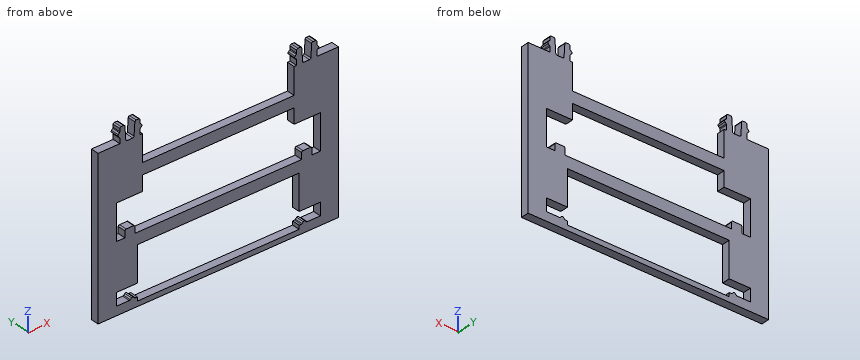
```python
from build123d import *

# Parameters (mm, degrees)
BOSS_EXTRUDE1_DEPTH = 1.6


with BuildPart() as part:
    # Sketch1 → Boss-Extrude1 (new body)
    with BuildSketch(Plane(origin=(0, 0, 0), x_dir=(1, 0, 0), z_dir=(0, 1, 0))):
        with BuildLine():
            Line((-68.929583289, 0), (-64.629583289, 0))
            Line((-64.629583289, 0), (-64.629583289, -0.996446609))
            ThreePointArc((-64.629583289, -0.996446609), (-64.648613406, -1.092117467), (-64.702806594, -1.173223305))
            Line((-64.702806594, -1.173223305), (-64.952806594, -1.423223305))
            ThreePointArc((-64.952806594, -1.423223305), (-65.026029899, -1.6), (-64.952806594, -1.776776695))
            Line((-64.952806594, -1.776776695), (-64.702806594, -2.026776695))
            ThreePointArc((-64.702806594, -2.026776695), (-64.648613406, -2.107882533), (-64.629583289, -2.203553391))
            Line((-64.629583289, -2.203553391), (-64.629583289, -2.75))
            ThreePointArc((-64.629583289, -2.75), (-64.556359984, -2.926776695), (-64.379583289, -3))
            Line((-64.379583289, -3), (-63.863471562, -3))
            ThreePointArc((-63.863471562, -3), (-63.692675541, -2.932561549), (-63.614025273, -2.766629753))
            Line((-63.614025273, -2.766629753), (-63.445141306, -0.233370247))
            ThreePointArc((-63.445141306, -0.233370247), (-63.366491038, -0.067438451), (-63.195695016, 0))
            Line((-63.195695016, 0), (-62.063471562, 0))
            ThreePointArc((-62.063471562, 0), (-61.892675541, -0.067438451), (-61.814025273, -0.233370247))
            Line((-61.814025273, -0.233370247), (-61.645141306, -2.766629753))
            ThreePointArc((-61.645141306, -2.766629753), (-61.566491038, -2.932561549), (-61.395695016, -3))
            Line((-61.395695016, -3), (-60.879583289, -3))
            ThreePointArc((-60.879583289, -3), (-60.702806594, -2.926776695), (-60.629583289, -2.75))
            Line((-60.629583289, -2.75), (-60.629583289, -2.203553391))
            ThreePointArc((-60.629583289, -2.203553391), (-60.610553172, -2.107882533), (-60.556359984, -2.026776695))
            Line((-60.556359984, -2.026776695), (-60.306359984, -1.776776695))
            ThreePointArc((-60.306359984, -1.776776695), (-60.23313668, -1.6), (-60.306359984, -1.423223305))
            Line((-60.306359984, -1.423223305), (-60.556359984, -1.173223305))
            ThreePointArc((-60.556359984, -1.173223305), (-60.610553172, -1.092117467), (-60.629583289, -0.996446609))
            Line((-60.629583289, -0.996446609), (-60.629583289, 0))
            Line((-60.629583289, 0), (-60.129583289, 0))
            Line((-60.129583289, 0), (-60.129583289, 5.25))
            Line((-60.129583289, 5.25), (-45.129583289, 5.25))
            Line((-45.129583289, 5.25), (-45.129583289, 7.5))
            Line((-45.129583289, 7.5), (-60.129583289, 7.5))
            Line((-60.129583289, 7.5), (-60.129583289, 10.5))
            Line((-60.129583289, 10.5), (-65.329583289, 10.5))
            Line((-65.329583289, 10.5), (-65.329583289, 17.5))
            Line((-65.329583289, 17.5), (-63.629583289, 17.5))
            Line((-63.629583289, 17.5), (-63.629583289, 16.25))
            ThreePointArc((-63.629583289, 16.25), (-63.556359984, 16.073223305), (-63.379583289, 16))
            Line((-63.379583289, 16), (-61.879583289, 16))
            ThreePointArc((-61.879583289, 16), (-61.702806594, 16.073223305), (-61.629583289, 16.25))
            Line((-61.629583289, 16.25), (-61.629583289, 17.5))
            Line((-61.629583289, 17.5), (-45.129583289, 17.5))
            Line((-45.129583289, 17.5), (-45.129583289, 19.75))
            Line((-45.129583289, 19.75), (-61.129583289, 19.75))
            Line((-61.129583289, 19.75), (-61.129583289, 26.75))
            Line((-61.129583289, 26.75), (-65.329583289, 26.75))
            Line((-65.329583289, 26.75), (-65.329583289, 29.25))
            Line((-65.329583289, 29.25), (-62.73313668, 29.25))
            ThreePointArc((-62.73313668, 29.25), (-62.637465822, 29.230969883), (-62.556359984, 29.176776695))
            Line((-62.556359984, 29.176776695), (-62.306359984, 28.926776695))
            ThreePointArc((-62.306359984, 28.926776695), (-62.129583289, 28.853553391), (-61.952806594, 28.926776695))
            Line((-61.952806594, 28.926776695), (-61.702806594, 29.176776695))
            ThreePointArc((-61.702806594, 29.176776695), (-61.621700757, 29.230969883), (-61.526029899, 29.25))
            Line((-61.526029899, 29.25), (-61.129583289, 29.25))
            Line((-61.129583289, 29.25), (-61.129583289, 30))
            Line((-61.129583289, 30), (-45.129583289, 30))
            Line((-45.129583289, 30), (-45.129583289, 31))
            Line((-45.129583289, 31), (-68.929583289, 31))
            Line((-68.929583289, 31), (-68.929583289, 20))
            Line((-68.929583289, 20), (-68.929583289, 0))
        make_face()
    boss_extrude1 = extrude(amount=BOSS_EXTRUDE1_DEPTH)

    # Mirror1: Boss-Extrude1 across plane
    add(boss_extrude1.mirror(Plane(origin=(-45.129583289, 1.6, -31), x_dir=(0, 0, 1), z_dir=(-1, 0, 0))))


solid = part.part
```
Can you work these out from the model? Positions are in its coordinate system, mm. Coordinates: 2 decimals unless noted, no trailing zeros. Loops run counter-clockwise (first coordinate to the right, second up) from the corner with the lowest first, then second, coordinate; pieces in that order, holes last. Notation, with made-up numbers: (38, 81) -> (80, 81) arc R17 cw to (80, 91) -> close; hole circle Ø10 at (-7, -6). An arc over 180 degrees is marked (long way). Answer as a JSON object with one key per item and string values.
1) Imagine slicing it at D-D (y = 0.6). Count the separate pieces of the cut face and the enclosed holes in it, then the cut area to 3 significant figures.
Results:
{"separate pieces": "1", "enclosed holes": "2", "area": "617 mm^2"}
2) Imagine slicing it at B-B (x = -44.5). Please give me the cut outline in (y, z), then the cut area to 3 significant figures.
Results:
{"outline": "(0, -31) -> (1.6, -31) -> (1.6, -30) -> (0, -30) -> close; (0, -19.75) -> (1.6, -19.75) -> (1.6, -17.5) -> (0, -17.5) -> close; (0, -7.5) -> (1.6, -7.5) -> (1.6, -5.25) -> (0, -5.25) -> close", "area": "8.80 mm^2"}
3) Imagine slicing it at C-C (z = -24.5). Please give me the cut outline in (x, y).
Results:
{"outline": "(-68.93, 0) -> (-61.13, 0) -> (-61.13, 1.6) -> (-68.93, 1.6) -> close; (-29.13, 0) -> (-21.33, 0) -> (-21.33, 1.6) -> (-29.13, 1.6) -> close"}
4) Imagine slicing it at A-A (z = -28). Please give me the cut outline in (x, y).
Results:
{"outline": "(-68.93, 0) -> (-65.33, 0) -> (-65.33, 1.6) -> (-68.93, 1.6) -> close; (-24.93, 0) -> (-21.33, 0) -> (-21.33, 1.6) -> (-24.93, 1.6) -> close"}
5) If I drill on line 1 (Z direction, x = -38, y = 0.2); line 2 (X direction, y = 0.6, z = -14.5); line 3 (X direction, y = 0.2, z = -0.5), over which ranges is the centre line in solid material (lowest first)?
Results:
{"line 1": "z = -31 to -30, -19.75 to -17.5, -7.5 to -5.25", "line 2": "x = -68.93 to -65.33, -24.93 to -21.33", "line 3": "x = -68.93 to -60.13, -30.13 to -21.33"}
6) For P1, Ø0.8, axis at x = -51, y = 1, coming from the +Z side; P2, Ø0.8, axis at y = 1, z = 0.5, coming from the +X side, each with a flat end and sliding along its axis, tell me the tip position at first contact or that it passes through.
Results:
{"P1": "stops at z = -5.25", "P2": "stops at x = -25.63"}
